CAD build for the part. Positions are in the model's coordinates, mm. Round coordinates to 2 decimals unless told otherwise and drop trailing zeros. Loops run counter-clockwise (first coordinate to the right, second up) from the corner with the lowest first, then second, coordinate; pieces in that order, holes last.
```python
from build123d import *

# Parameters (mm, degrees)
F0_R         = 11
F1_DEPTH     = 3
F2_T2_ANGLE  = 120
F2_T4_ANGLE  = 240
F2_T6_ANGLE  = 240
F2_T8_ANGLE  = 120
F2_T10_ANGLE = 240
F2_T12_ANGLE = 120


# Not quite as in the source:
# - a fillet or chamfer that OpenCascade refuses, or shapes differently, is made with other operations: its cross-section is extruded or revolved along the edge and cut away or added


with BuildPart() as f1:
    # F0 (on Top) → F1 (new body)
    with BuildSketch(Plane.XY):
        with BuildLine():
            ThreePointArc((12.9903810568, 22.5), (14.4888873943, 26.1177143235), (15, 30))
            ThreePointArc((15, 30), (-3.8822856765, 44.4888873943), (-12.9903810568, 22.5))
            ThreePointArc((-12.9903810568, 22.5), (0, 15), (12.9903810568, 22.5))
        make_face()
        with Locations((0, 30)):
            Circle(F0_R, mode=Mode.SUBTRACT)
        with BuildLine():
            ThreePointArc((12.9903810568, 22.5), (0, 15), (-12.9903810568, 22.5))
            ThreePointArc((-12.9903810568, 22.5), (-12.9903810568, 7.5), (-25.9807621135, 0))
            ThreePointArc((-25.9807621135, 0), (-15.3741603957, -4.3933982822), (-10.9807621135, -15))
            ThreePointArc((-10.9807621135, -15), (-11.4918747192, -18.8822856765), (-12.9903810568, -22.5))
            ThreePointArc((-12.9903810568, -22.5), (0, -15), (12.9903810568, -22.5))
            ThreePointArc((12.9903810568, -22.5), (12.9903810568, -7.5), (25.9807621135, 0))
            ThreePointArc((25.9807621135, 0), (12.9903810568, 7.5), (12.9903810568, 22.5))
        make_face()
        Circle(F0_R, mode=Mode.SUBTRACT)
        with BuildLine():
            ThreePointArc((-10.9807621135, -15), (-15.3741603957, -4.3933982822), (-25.9807621135, 0))
            ThreePointArc((-25.9807621135, 0), (-38.9711431703, -22.5), (-12.9903810568, -22.5))
            ThreePointArc((-12.9903810568, -22.5), (-11.4918747192, -18.8822856765), (-10.9807621135, -15))
        make_face()
        with Locations((-25.9807621135, -15)):
            Circle(F0_R, mode=Mode.SUBTRACT)
        with BuildLine():
            ThreePointArc((40.9807621135, -15), (36.5873638313, -4.3933982822), (25.9807621135, 0))
            ThreePointArc((25.9807621135, 0), (12.9903810568, -7.5), (12.9903810568, -22.5))
            ThreePointArc((12.9903810568, -22.5), (29.8630477901, -29.4888873943), (40.9807621135, -15))
        make_face()
        with Locations((25.9807621135, -15)):
            Circle(F0_R, mode=Mode.SUBTRACT)
    extrude(amount=F1_DEPTH)

    # F2: fillet of radius 4 on 1 edges, made by hand

    # F2_s1 → F2_t2 (revolve, cut)
    with BuildSketch(Plane(origin=(-12.9903810568, 22.5, 0), x_dir=(0, 0, 1), z_dir=(-0.5, 0.8660254038, 0))):
        with BuildLine():
            ThreePointArc((0, 0), (2.1622776602, 1.4234936034), (3, 3.8729833462))
            Line((3, 3.8729833462), (3, 0))
            Line((3, 0), (0, 0))
        make_face()
    revolve(axis=Axis((-25.9807621135, 15, 3), (0, 0, -1)), revolution_arc=F2_T2_ANGLE, mode=Mode.SUBTRACT)

    # F2_s3 → F2_t4 (revolve, cut)
    with BuildSketch(Plane(origin=(12.9903810568, 22.5, 0), x_dir=(0, 0, 1), z_dir=(-0.5, -0.8660254038, 0))):
        with BuildLine():
            ThreePointArc((0, 0), (2.1622776602, 1.4234936034), (3, 3.8729833462))
            Line((3, 3.8729833462), (3, 0))
            Line((3, 0), (0, 0))
        make_face()
    revolve(axis=Axis((0, 30, 3), (0, 0, 1)), revolution_arc=F2_T4_ANGLE, mode=Mode.SUBTRACT)

    # F2_s5 → F2_t6 (revolve, cut)
    with BuildSketch(Plane.YZ.offset(-25.9807621135)):
        with BuildLine():
            ThreePointArc((0, 0), (-1.4234936034, 2.1622776602), (-3.8729833462, 3))
            Line((-3.8729833462, 3), (0, 3))
            Line((0, 3), (0, 0))
        make_face()
    revolve(axis=Axis((-25.9807621135, -15, 3), (0, 0, 1)), revolution_arc=F2_T6_ANGLE, mode=Mode.SUBTRACT)

    # F2_s7 → F2_t8 (revolve, cut)
    with BuildSketch(Plane(origin=(-12.9903810568, -22.5, 0), x_dir=(0, 0, 1), z_dir=(-0.5, -0.8660254038, 0))):
        with BuildLine():
            ThreePointArc((0, 0), (2.1622776602, 1.4234936034), (3, 3.8729833462))
            Line((3, 3.8729833462), (3, 0))
            Line((3, 0), (0, 0))
        make_face()
    revolve(axis=Axis((0, -30, 3), (0, 0, -1)), revolution_arc=F2_T8_ANGLE, mode=Mode.SUBTRACT)

    # F2_s9 → F2_t10 (revolve, cut)
    with BuildSketch(Plane(origin=(12.9903810568, -22.5, 0), x_dir=(0, 0, 1), z_dir=(-0.5, 0.8660254038, 0))):
        with BuildLine():
            ThreePointArc((0, 0), (2.1622776602, 1.4234936034), (3, 3.8729833462))
            Line((3, 3.8729833462), (3, 0))
            Line((3, 0), (0, 0))
        make_face()
    revolve(axis=Axis((25.9807621135, -15, 3), (0, 0, 1)), revolution_arc=F2_T10_ANGLE, mode=Mode.SUBTRACT)

    # F2_s11 → F2_t12 (revolve, cut)
    with BuildSketch(Plane.YZ.offset(25.9807621135)):
        with BuildLine():
            ThreePointArc((0, 0), (-1.4234936034, 2.1622776602), (-3.8729833462, 3))
            Line((-3.8729833462, 3), (0, 3))
            Line((0, 3), (0, 0))
        make_face()
    revolve(axis=Axis((25.9807621135, 15, 3), (0, 0, -1)), revolution_arc=F2_T12_ANGLE, mode=Mode.SUBTRACT)


solid = f1.part
```
Item 1: Cut at A-A, the plane x = 0. Give the cut face in (y, z), plus the area to 3 significant figures.
Answers follow:
outline: (-15, 0) - (-11, 0) - (-11, 3) - (-11.13, 3) arc R4 ccw to start; (11, 0) - (19, 0) - (19, 3) - (11, 3) - close; (41, 0) - (45, 0) arc R4 ccw to (41.13, 3) - (41, 3) - close
area: 42.0 mm2
Item 2: Cut at D-D, the plane y = -23.5. State how many separate pieces and enclosed holes the cut face has, plus the area to 3 significant figures.
Answers follow:
separate pieces: 4
enclosed holes: 0
area: 49.4 mm2
Item 3: Cut at C-C, the plane z = 1.7. Give the cut face in (x, y), plus the area to 3 significant figures.
Answers follow:
outline: (-25.98, -0.92) arc R14.08 ccw (long way) to (-13.79, -22.04) arc R15.92 cw to (13.79, -22.04) arc R14.08 ccw (long way) to (25.98, -0.92) arc R15.92 cw to (12.19, 22.96) arc R14.08 ccw (long way) to (-12.19, 22.96) arc R15.92 cw to start; hole circle Ø22 at (-25.98, -15); hole circle Ø22 at (0, 0); hole circle Ø22 at (0, 30); hole circle Ø22 at (25.98, -15)
area: 1,270 mm2
Item 4: Flat gauge pins, fed straight in: P1, Ø1, axis at x = -18.5, z = 2.5, coming from the -Y side; P2, Ø1.5, axis at x = 29.5, y = -22.5, coming from the -Z side; P3, Ø5, axis at x = -13, y = 35.5, coming from the -Z side; P4, Ø1, axis at y = 26.5, z = 1.5, coming from the +X side. Where does each tip first touch, or does it go through?
Answers follow:
P1: stops at y = -26.63
P2: passes through
P3: stops at z = 0
P4: stops at x = 14.19
Item 5: Probe line 1 (Y direction, x = 0, z = 1.9); line 2 (Y direction, x = 6, z = 2.1); line 3 (Y direction, x = 27.5, z = 1.1). List the from-to ranges inside material, lowest first.
Answers follow:
line 1: y = -13.88 to -11, 11 to 19, 41 to 43.88
line 2: y = -14.8 to -9.22, 9.22 to 20.78, 39.22 to 42.27
line 3: y = -29.45 to -25.89, -4.11 to -0.55
Item 6: Cut at B-B, the plane y = 30. Give the cut face in (x, z), plus the area to 3 significant figures.
Answers follow:
outline: (-15, 0) - (-11, 0) - (-11, 3) - (-11.13, 3) arc R4 ccw to start; (11, 0) - (15, 0) arc R4 ccw to (11.13, 3) - (11, 3) - close
area: 18.0 mm2
